```python
from build123d import *

# Parameters (mm, degrees)
SKETCH2_R               = 3
SKETCH2_R_2             = 2.5
BOSS_EXTRUDE1_DEPTH     = 6.35
SKETCH3_W               = 7.9375
SKETCH3_H               = 3.175
CUT_EXTRUDE1_DEPTH      = 1
CUT_EXTRUDE1_DEPTH_BACK = 521.7


with BuildPart() as part:
    # Sketch2 → Boss-Extrude1 (new body)
    with BuildSketch(Plane(origin=(0, 0, 0), x_dir=(1, 0, 0), z_dir=(0, 1, 0))):
        Polygon((0, 0), (0, 182.5625), (41.275, 520.7), (74.6125, 520.7), (207.9625, 177.8), (207.9625, 0), align=None)
        with Locations((60.061658842, 504.825)):
            Circle(SKETCH2_R, mode=Mode.SUBTRACT)
        with Locations((20.301658842, 190.035)):
            Circle(SKETCH2_R_2, mode=Mode.SUBTRACT)
        with Locations((190.081658842, 189.735)):
            Circle(SKETCH2_R_2, mode=Mode.SUBTRACT)
        with Locations((190.001658842, 19.755)):
            Circle(SKETCH2_R_2, mode=Mode.SUBTRACT)
        with Locations((90.031658842, 19.755)):
            Circle(SKETCH2_R_2, mode=Mode.SUBTRACT)
        with Locations((60.061658842, 159.795)):
            Circle(SKETCH2_R, mode=Mode.SUBTRACT)
    extrude(amount=BOSS_EXTRUDE1_DEPTH)

    # Sketch3 → Cut-Extrude1 (cut, two sides)
    with BuildSketch(Plane.XY) as cut_extrude1_sk:
        with Locations((3.96875, 4.7625)):
            Rectangle(SKETCH3_W, SKETCH3_H)
        with Locations((203.99375, 4.7625)):
            Rectangle(SKETCH3_W, SKETCH3_H)
    extrude(amount=CUT_EXTRUDE1_DEPTH, mode=Mode.SUBTRACT)
    extrude(cut_extrude1_sk.sketch, amount=-CUT_EXTRUDE1_DEPTH_BACK, mode=Mode.SUBTRACT)


solid = part.part
```
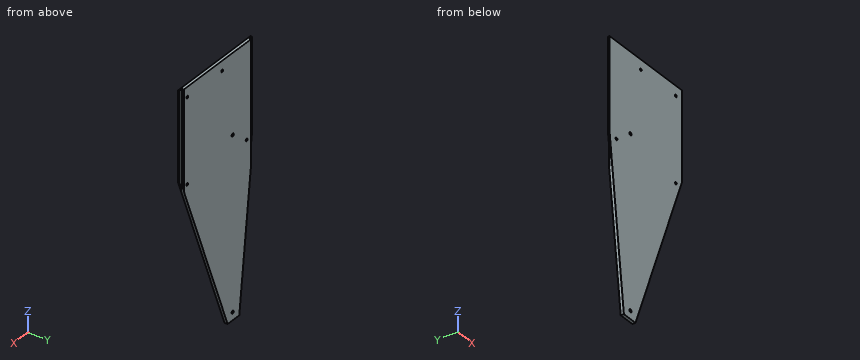
Part model, mm, in its own coordinate system. Coordinates: 2 decimals unless noted, no trailing zeros. Loops run counter-clockwise (first coordinate to the right, second up) from the corner with the lowest first, then second, coordinate; pieces in that order, holes last. Notation, with made-up numbers: (6, -16.75) - (64, -16.75) arc R24 cw to (64, 21.25) - close; hole circle Ø8 at (-0.75, -12). An arc over 180 degrees is marked (long way). Write item = value, one per line. Start each with the question number.
Item 1: Flat gauge pins, fed straight in: pin 1 Ø4 at (x, z) = (2, -170) entering from +Y (3 decimals); pin 2 Ø1 at (y, z) = (1, -197.5) entering from +X; pin 3 Ø1.6 at (y, z) = (5, -100.5) entering from +X (3 decimals); pin 4 Ø3 at (x, z) = (190, -19.76) entering from -Y. Where does each tip first touch, or does it go through?
Item 2: Cut at B-B, the plane y = 4.75. Give the cut face in (x, z) (1 decimal).
Item 3: Wall check: L1, parallel to Z at x = 58.5, y = 5.25; L2, parallel to X at y = 4.75, z = -166.5 (1 decimal); L3, parallel to X at y = 1.25, z = -192. Give the ranges that are in metal, low to high. Write a range as from..to.
Item 4: Cut at C-C, the plane x = 140. Give the cut face in (y, z).
The answers:
q1.pin_1 = 3.175
q1.pin_2 = 200.5
q1.pin_3 = 200.025
q1.pin_4 = through
q2.outline = (7.9, -247.6) - (41.3, -520.7) - (74.6, -520.7) - (200, -198.2) - (200, 0) - (7.9, 0) - close; hole circle Ø5 at (20.3, -190); hole circle Ø6 at (60.1, -504.8); hole circle Ø6 at (60.1, -159.8); hole circle Ø5 at (90, -19.8); hole circle Ø5 at (190, -19.8); hole circle Ø5 at (190.1, -189.7)
q3.L1 = -520.7..-507.39, -502.26..-162.36, -157.23..0
q3.L2 = 7.9..200
q3.L3 = 1.15..18.76, 21.85..189.02, 191.14..202.44
q4.outline = (0, -352.56) - (6.35, -352.56) - (6.35, 0) - (0, 0) - close
